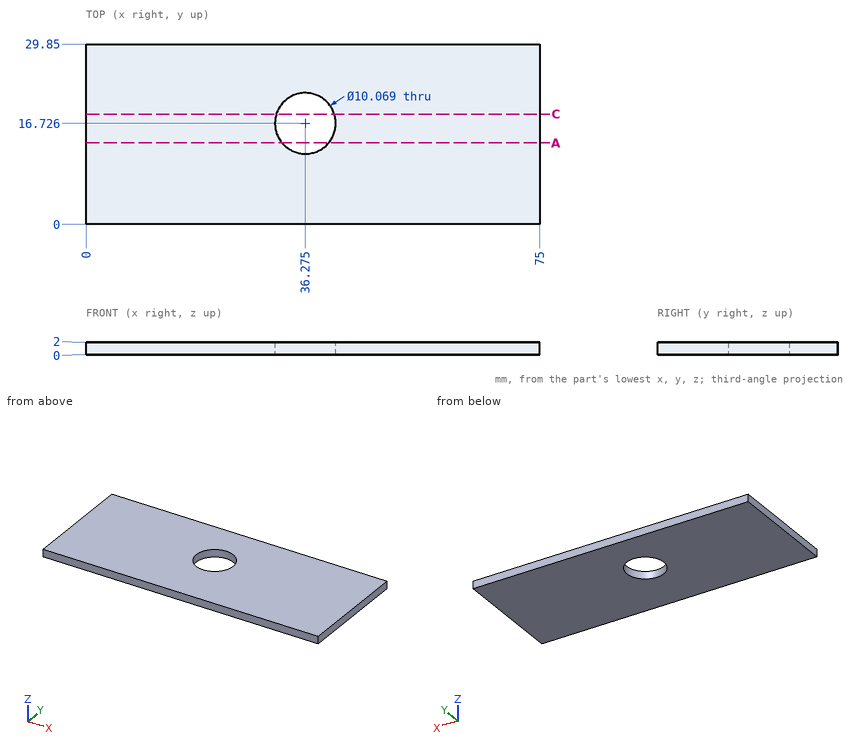
Geometry check sheet. Reference: drawing and pictorial views, mm from the part's lowest x, y, z. Round coordinates to 2 decimals unless told otherwise and drop trailing zeros. Order: outer loops, then holes, each group sorted by start corner. A loop starts at its lowest first (then second) coordinate and runs counter-clockwise, first axis right, second up. Notation, with made-up numbers: (-4.75, 74.25) - (19.25, 74.25) arc R19 cw to (19.25, 89.25) - close; hole circle Ø9 at (17.25, 80). An arc over 180 degrees is marked (long way). Use a Markdown table: item, result. Add a question column.
1) Section check A-A (y = 13.5). Record the cut outline in (x, z).
2) Section check C-C (y = 18.25). Record the cut outline in (x, z), then the cut area to 3 significant figures.
3) Thickness scan on line 1 along X through (y, z) = (14.75, 0.7) (1 decimal); line 2 along X through (y, z) = (13.25, 1.15) (1 decimal). Record the ranges inside material, lowest first.
Established:
| question | item | result |
|---|---|---|
| 1 | outline | (0, 0) - (32.41, 0) - (32.41, 2) - (0, 2) - close; (40.14, 0) - (75, 0) - (75, 2) - (40.14, 2) - close |
| 2 | outline | (0, 0) - (31.48, 0) - (31.48, 2) - (0, 2) - close; (41.07, 0) - (75, 0) - (75, 2) - (41.07, 2) - close |
| 2 | area | 131 mm2 |
| 3 | line 1 | 0 to 31.6, 40.9 to 75 |
| 3 | line 2 | 0 to 32.6, 39.9 to 75 |
